Check sheet for the modelled part. Datum: model origin and axes. Units: mm. A direction names the side the tool comes from. Round coordinates to 2 decimals unless told otherwise and drop trailing zeros. Loops run counter-clockwise (first coordinate to the right, second up) from the corner with the lowest first, then second, coordinate; pieces in that order, holes last. Notation, with made-up numbers: (85, 11) - (138, 11) arc R25 cw to (138, 48) - close; hole circle Ø5 at (26.5, 46.5). An arc over 180 degrees is marked (long way). Answer in a Markdown table with one row per item. Add a question column.
(1) Cross-section at D-D on z = -212.7. Enter the section's corners in (x, y).
(2) Cross-section at C-C on y = 50. Enter the section's corners in (x, z), then the cut area to 3 significant figures.
(3) Gauge pin test, flat ends, axial feed: pin 1 (4 mm diameter, centred on y = 49, z = -128.5, fed in from -X); pin 2 (6.5 mm diameter, centred on y = 25.98, z = -236.72, fed in from +X); pin 3 (5.5 mm diameter, centred on y = 72.22, z = -328.12, fed in from -X). Record the tip position at first contact, or that the pin passes through.
(4) Cross-section at A-A on x = -20. Enter the section's corners in (y, z), then the cut area to 3 significant figures.
(5) Cross-section at B-B on z = -435. Enter the section's corners in (x, y).
(6) Access from +Z, -Z, +X, -X, +Y, -Y to the whole of each face (thin tool, end or side, straight path). Record for faces 5 (the cylindrical face through (-15.386, 41.128, -10.14)), 6 (the cylindrical face through (62.605, 27.181, -192.494)), 7 (the flat face through (50, 49, -230)).
(7) Thickness scan on line 1 along Y through (x, z) = (60, -212); line 2 along X through (y, z) = (50, -13.25); line 3 along Y through (x, z) = (54.5, -435). Record the ranges inside material, lowest first.
(8) Mould release check, pull along Y, two halves, no side actions. Record for faces 1 (the flat face through (59, 0, -177)), 2 (the flat face through (11, 49, 0)), 3 (the flat face through (55, 26, -189)), 4 (the flat face through (59, 100, -177)): +Y half, -Y half, draft (parallel to the pull), parting line (faces both ways), or undercut.
from build123d import *

# Parameters (mm, degrees)
BOSS_EXTRUDE1_DEPTH     = 100
CUT_EXTRUDE2_DEPTH      = 467.261729075
CUT_EXTRUDE2_DEPTH_BACK = 467.261729075
SKETCH4_R               = 10
FILLET1_R               = 5
SKETCH5_R               = 4
CUT_EXTRUDE3_DEPTH      = 15
SKETCH6_R               = 4
CUT_EXTRUDE4_DEPTH      = 20
SKETCH7_R               = 3
CUT_EXTRUDE5_DEPTH      = 13


with BuildPart() as part:
    # Sketch1 → Boss-Extrude1 (new body)
    with BuildSketch(Plane(origin=(0, 0, 0), x_dir=(1, 0, 0), z_dir=(0, 1, 0))):
        Polygon((50, 20), (50, 450), (70, 450), (70, 0), (-50, 0), (-50, 20), align=None)
    extrude(amount=BOSS_EXTRUDE1_DEPTH)

    # Sketch4 → Cut-Extrude2 (cut, two sides: drawn at the far end of the back side and taken through both)
    with BuildSketch(Plane.XY.offset(-CUT_EXTRUDE2_DEPTH_BACK)):
        with Locations((-20, 50)):
            Circle(SKETCH4_R)
    extrude(amount=CUT_EXTRUDE2_DEPTH + CUT_EXTRUDE2_DEPTH_BACK, mode=Mode.SUBTRACT)

    # Fillet1
    fillet1_edges = [part.edges().sort_by_distance(p)[0] for p in [
        (-50, 50, 0),
        (-50, 50, -20),
        (50, 50, -450),
        (70, 50, -450),
        (70, 50, 0),
        (60, 100, -450),
        (50, 100, -235),
        (0, 100, -20),
        (-50, 100, -10),
        (10, 100, 0),
        (-50, 0, -10),
        (0, 0, -20),
        (50, 0, -235),
        (60, 0, -450),
        (70, 0, -225),
        (10, 0, 0),
        (70, 100, -225),
    ]]
    fillet(fillet1_edges, radius=FILLET1_R)

    # Sketch5 → Cut-Extrude3 (cut)
    with BuildSketch(Plane(origin=(70, 0, 0), x_dir=(0, 0, -1), z_dir=(1, 0, 0))):
        with Locations((212.7, 83.970575503)):
            Circle(SKETCH5_R)
        with Locations((236.720824299, 74.020824299)):
            Circle(SKETCH5_R)
        with Locations((246.670575503, 50)):
            Circle(SKETCH5_R)
        with Locations((236.720824299, 25.979175701)):
            Circle(SKETCH5_R)
        with Locations((212.7, 16.029424497)):
            Circle(SKETCH5_R)
        with Locations((188.679175701, 25.979175701)):
            Circle(SKETCH5_R)
        with Locations((178.729424497, 50)):
            Circle(SKETCH5_R)
        with Locations((188.679175701, 74.020824299)):
            Circle(SKETCH5_R)
    extrude(amount=-CUT_EXTRUDE3_DEPTH, mode=Mode.SUBTRACT)

    # Sketch6 → Cut-Extrude4 (cut)
    with BuildSketch(Plane(origin=(70, 0, 0), x_dir=(0, 0, -1), z_dir=(1, 0, 0))):
        with Locations((395, 10)):
            Circle(SKETCH6_R)
        with Locations((435, 10)):
            Circle(SKETCH6_R)
        with Locations((435, 90)):
            Circle(SKETCH6_R)
        with Locations((395, 90)):
            Circle(SKETCH6_R)
    extrude(amount=-CUT_EXTRUDE4_DEPTH, mode=Mode.SUBTRACT)

    # Sketch7 → Cut-Extrude5 (cut)
    with BuildSketch(Plane.ZY.offset(-50)):
        with Locations((-363.04375, 72.225)):
            Circle(SKETCH7_R)
        with Locations((-328.11875, 72.225)):
            Circle(SKETCH7_R)
        with Locations((-363.04375, 27.775)):
            Circle(SKETCH7_R)
        with Locations((-328.11875, 27.775)):
            Circle(SKETCH7_R)
    extrude(amount=-CUT_EXTRUDE5_DEPTH, mode=Mode.SUBTRACT)


solid = part.part
Answers:
| question | item | result |
|---|---|---|
| 1 | outline | (50, 5) arc R5 ccw to (55, 0) - (65, 0) arc R5 ccw to (70, 5) - (70, 12.03) - (55, 12.03) - (55, 20.03) - (70, 20.03) - (70, 79.97) - (55, 79.97) - (55, 87.97) - (70, 87.97) - (70, 95) arc R5 ccw to (65, 100) - (55, 100) arc R5 ccw to (50, 95) - close |
| 2 | outline | (-50, -15) arc R5 ccw to (-45, -20) - (-30, -20) - (-30, 0) - (-45, 0) arc R5 ccw to (-50, -5) - close; (-10, -20) - (50, -20) - (50, -445) arc R5 ccw to (55, -450) - (65, -450) arc R5 ccw to (70, -445) - (70, -250.67) - (55, -250.67) - (55, -242.67) - (70, -242.67) - (70, -182.73) - (55, -182.73) - (55, -174.73) - (70, -174.73) - (70, -5) arc R5 ccw to (65, 0) - (-10, 0) - close |
| 2 | area | 10,300 mm^2 |
| 3 | pin 1 | stops at x = 50 |
| 3 | pin 2 | stops at x = 55 |
| 3 | pin 3 | stops at x = 63 |
| 4 | outline | (0, -15) arc R5 ccw to (5, -20) - (40, -20) - (40, 0) - (5, 0) arc R5 ccw to (0, -5) - close; (60, -20) - (95, -20) arc R5 ccw to (100, -15) - (100, -5) arc R5 ccw to (95, 0) - (60, 0) - close |
| 4 | area | 1,580 mm^2 |
| 5 | outline | (50, 5) arc R5 ccw to (55, 0) - (65, 0) arc R5 ccw to (70, 5) - (70, 6) - (50, 6) - close; (50, 14) - (70, 14) - (70, 86) - (50, 86) - close; (50, 94) - (70, 94) - (70, 95) arc R5 ccw to (65, 100) - (55, 100) arc R5 ccw to (50, 95) - close |
| 6 | face 5 | +Z, -Z |
| 6 | face 6 | +X |
| 6 | face 7 | -Z, -X, +Y, -Y |
| 7 | line 1 | y = 0 to 12.09, 19.97 to 80.03, 87.91 to 100 |
| 7 | line 2 | x = -50 to -30, -10 to 70 |
| 7 | line 3 | y = 0.03 to 6, 14 to 86, 94 to 99.97 |
| 8 | face 1 | -Y half |
| 8 | face 2 | draft |
| 8 | face 3 | undercut |
| 8 | face 4 | +Y half |
